Autodesk Inventor part; units mm, degrees
ref_plane "Work Plane2" through (0, 0, 55) normal (0.9994, 0, 0.0349) x (0, 1, 0)
ref_plane "YZ Plane" through (0, 0, 0) normal (1, 0, 0) x (0, 1, 0)
ref_plane "XZ Plane" through (0, 0, 0) normal (0, 1, 0) x (-1, 0, 0)
sketch "Sketch24" plane through (0, 0, 0) normal (0, 1, 0) x (-1, 0, 0)
  line L0 (0, 0) -> (90, 0)
  line L1 (90, 0) -> (90, 55)
  line L2 (90, 55) -> (0, 55)
  line L3 (0, 55) -> (0, 0)
  dimension "d160" = 55
  dimension "d161" = 90
extrude "Extrusion21" add sketch "Sketch24" along normal blind 17
sketch "Sketch25" plane through (0, 0, 0) normal (0, -1, 0) x (1, 0, 0)
  circle A0 centre (-70, 50) radius 2.5
  circle A1 centre (-35, 5) radius 2.5
  line L0 (0, 0) -> (-90, 0)
  line L1 (-90, 55) -> (0, 55)
  line L2 (-90, 0) -> (-90, 55)
  dimension "d164" = 5
  dimension "d165" = 5
  dimension "d166" = 5
  dimension "d167" = 5
  dimension "d168" = 20
  dimension "d169" = 55
extrude "Extrusion22" cut sketch "Sketch25" against normal blind 14
sketch "Sketch26" plane through (0, 17, 0) normal (0, 1, 0) x (1, 0, 0)
  line L0 (-63.0815, -3.8119) -> (-26.3119, -40.5815)
  line L1 (-26.3119, -40.5815) -> (-36.9185, -51.1881)
  line L2 (-36.9185, -51.1881) -> (-73.6881, -14.4185)
  line L3 (-73.6881, -14.4185) -> (-63.0815, -3.8119)
  line L4 (-90, 0) -> (-90, -55)
  line L5 (0, 0) -> (-90, 0)
  point P0 (0, -22.5)
  dimension "d172" = 15
  dimension "d173" = 52
  dimension "d176" = 47.3762
  dimension "d177" = 47.3762
  dimension "d181" = 16.3119
  dimension "d182" = 45
  dimension "d183" = 3.8119
extrude "Extrusion23" cut sketch "Sketch26" against normal through all
ref_plane "Work Plane2" through (0, 0, 55) normal (0.9994, 0, 0.0349) x (0, 1, 0)
sketch "Sketch28" plane through (0, 0, 55) normal (0.9994, 0, 0.0349) x (0, 1, 0)
  circle A0 centre (27, -25.9665) radius 22.5
  line L0 (17, 0) -> (17, -54.9665)
  line L1 (0, -54.9665) -> (17, -54.9665)
  line L2 (0, 0) -> (0, -54.9665)
  dimension "d187" = 45
  dimension "d192" = 29
  dimension "d194" = 27
extrude "Extrusion24" cut sketch "Sketch28" against normal through all
sketch "Sketch29" plane through (0, 17, 0) normal (0, 1, 0) x (1, 0, 0)
  line L0 (-26.3119, -40.5815) -> (-63.0815, -3.8119)
  line L1 (-44.6967, -22.1967) -> (-55.3033, -32.8033)
  line L2 (-73.6881, -14.4185) -> (-40.3293, -47.7773)
  arc A0 (-68.4344, -7.51) -> (-69.99, -9.0656) centre (-70.0818, -7.4182) ccw
  line L3 (-63.5547, -12.3896) -> (-68.4344, -7.51)
  line L4 (-69.99, -9.0656) -> (-65.1104, -13.9453)
  line L5 (-65.1104, -13.9453) -> (-63.5547, -12.3896)
  line L6 (-65.8208, -6.5512) -> (-63.0815, -3.8119)
  arc A1 (-31.5656, -47.49) -> (-30.01, -45.9344) centre (-29.9182, -47.5818) ccw
  line L7 (-34.8896, -41.0547) -> (-30.01, -45.9344)
  line L8 (-31.5656, -47.49) -> (-36.4453, -42.6104)
  line L9 (-36.4453, -42.6104) -> (-34.8896, -41.0547)
  line L10 (-29.0512, -43.3208) -> (-26.3119, -40.5815)
  point P0 (0, 0)
  point P1 (-73.6881, -14.4185)
  point P2 (-56.553, -49.6596)
  point P3 (-21.3119, -14.4185)
  point P4 (-40.3293, -47.7773)
  point P5 (-36.9185, -51.1881)
  dimension "d216" = 2.2
  dimension "d217" = 1.1
  dimension "d218" = 3.3
  dimension "d219" = 2.4
  dimension "d221" = 7.5
  dimension "d222" = 15
extrude "Extrusion25" cut sketch "Sketch29" against normal blind 10.5
fillet "Fillet4" radius 2 4 edges at (-26.3119, 4.1375, 40.5815) (-63.0815, 8.5, 3.8119) (-73.6881, 3.9894, 14.4185) (-36.9185, 8.5, 51.1881)
sketch "Sketch31" plane through (0, 0, 0) normal (0, -1, 0) x (1, 0, 0)
  line L0 (7.4187, -6.4354) -> (-15, -6.4354)
  line L1 (-15, -6.4354) -> (-15, 10)
  line L2 (-15, 10) -> (7.4187, 10)
  line L3 (7.4187, 10) -> (7.4187, -6.4354)
  line L4 (0, 55) -> (0, 0)
  line L5 (0, 0) -> (-90, 0)
  line L6 (0, 0) -> (-90, 0)
  line L7 (-90, 55) -> (0, 55)
  line L8 (0, 27.5) -> (-90, 27.5)
  line L9 (-45, 62.4242) -> (-45, -8.4375)
  line L10 (-90, 0) -> (-90, 55)
  line L11 (7.4187, 61.4354) -> (-15, 61.4354)
  line L12 (-15, 61.4354) -> (-15, 45)
  line L13 (-15, 45) -> (7.4187, 45)
  line L14 (7.4187, 45) -> (7.4187, 61.4354)
  line L15 (-97.4187, -6.4354) -> (-75, -6.4354)
  line L16 (-75, -6.4354) -> (-75, 10)
  line L17 (-75, 10) -> (-97.4187, 10)
  line L18 (-97.4187, 10) -> (-97.4187, -6.4354)
  line L19 (-90, 55) -> (-90, 0)
  line L20 (-97.4187, 61.4354) -> (-75, 61.4354)
  line L21 (-75, 61.4354) -> (-75, 45)
  line L22 (-75, 45) -> (-97.4187, 45)
  line L23 (-97.4187, 45) -> (-97.4187, 61.4354)
  point P0 (-17, 0)
  point P1 (-17, 55)
  point P2 (-73, 0)
  point P3 (-73, 55)
  dimension "d227" = 15
  dimension "d228" = 10
  dimension "d229" = 45
  dimension "d230" = 90
extrude "Extrusion27" cut sketch "Sketch31" against normal through all contours L0 L1 L5 L4 L2 L3 | L1 L2 L4 L5 | L16 L15 L18 L17 L10 L5 | L5 L10 L17 L16 | L13 L12 L7 L4 | L4 L7 L12 L11 L14 L13 | L22 L23 L20 L21 L7 L10 | L10 L7 L21 L22
fillet "Fillet5" radius 2 4 edges at (-15, 7.0843, 10) (-75, 5.7918, 10) (-75, 7.1624, 45) (-15, 5.8494, 45)
sketch "Sketch32" plane through (0, 0, 45) normal (0, 0, 1) x (1, 0, 0)
  line L0 (0, 0) -> (-24.7878, 29.541)
  line L1 (-24.7878, 29.541) -> (8.6873, 22.432)
  line L2 (8.6873, 22.432) -> (0, 0)
  line L3 (0, 0) -> (-13, 0)
  dimension "d234" = 50
extrude "Extrusion28" cut sketch "Sketch32" against normal through all
properties part number "GuideCarotte" material "Nylon 6/6"
Check sheet for the modelled part. Datum: model origin and axes. Units: mm. A direction names the side the tool comes from. Give positions to 0.01 mm unless a question says otherwise; leave off trailing zeros. Write each loop counter-clockwise with the first axis right and the second up, starting at its lowest first coordinate (ties: lowest second). Pieces come first, ordered by that corner, then holes. Notation, with made-up numbers: (88, -27) -> (112, -27) arc R13 ccw to (112, -5) -> close; hole circle Ø8 at (4.25, 16). An arc over 180 degrees is marked (long way). One line per item, written item: value. Start each with the question number.
Item 1: Material ranges on probe 1 along Z at (x, y) = (-36, 11.75); probe 2 along Z at (x, y) = (-35, 7.5); probe 3 along X at (y, z) = (1.75, 24), recorded low to high. Write a range as from..to.
Item 2: Section check A-A on y = 3.25. Record the cut outline in (x, z).
Item 3: Tool access check on faces 4 (the flat face through (-75, 8, 51)), 5 (the cylindrical face through (-25.38, 5.1, 22.97)), 6 (the flat face through (-15, 8, 4)), 7 (the cylindrical face through (-63.1, 8.38, 4.64)). Record the directions out of +Z, -Z, +X, -X, +Y, -Y that give a thin tool (end or side, any length) a straight path to the whole face; none if there is none.
Item 4: Draft check along Z on faces 1 (the flat face through (-66.71, 6.73, 7.44)), 2 (the cylindrical face through (-14.43, 8.62, 9.4)), 3 (the flat face through (-15, 8, 51)). Enter one of: +Z half, -Z half, draft (parallel to the pull), parting line (faces both ways), or undercut.
Item 5: Gauge pin test, flat ends, axial feed: pin 1 (3.5 mm diameter, centred on x = -4.5, y = 8, fed in from +Z); pin 2 (3 mm diameter, centred on y = 15, z = 42, fed in from -X); pin 3 (3.5 mm diameter, centred on x = -86.5, y = 4.5, fed in from -Z); pin 4 (2 mm diameter, centred on x = -70, z = 7, fed in from +Y). Record the tip position at first contact, or that the pin passes through.
Results list:
1. probe 1: 0..2.71, 7.29..11.21, 50.14..55
1. probe 2: 0..2.5, 7.5..16.56, 49.27..55
1. probe 3: -90..-64.11, -42.89..-1.47
2. outline: (-90, 10) -> (-77, 10) arc R2 cw to (-75, 8) -> (-75, 0) -> (-15, 0) -> (-15, 8) arc R2 cw to (-13, 10) -> (-2.73, 10) -> (-2.73, 45) -> (-13, 45) arc R2 cw to (-15, 47) -> (-15, 55) -> (-75, 55) -> (-75, 47) arc R2 cw to (-77, 45) -> (-90, 45) -> close; hole circle Ø5 at (-70, 50); hole (-72.27, 13) -> (-64.5, 5.23) arc R2 ccw to (-61.67, 5.23) -> (-27.73, 39.17) arc R2 ccw to (-27.73, 42) -> (-35.5, 49.77) arc R2 ccw to (-38.33, 49.77) -> (-72.27, 15.83) arc R2 ccw to start; hole circle Ø5 at (-35, 5)
3. face 4: +Z, -X, +Y, -Y
3. face 5: +Y
3. face 6: -Z, +X, +Y, -Y
3. face 7: +Y, -Y
4. face 1: undercut
4. face 2: -Z half
4. face 3: draft
5. pin 1: z = 45
5. pin 2: through
5. pin 3: z = 10
5. pin 4: y = 6.5
